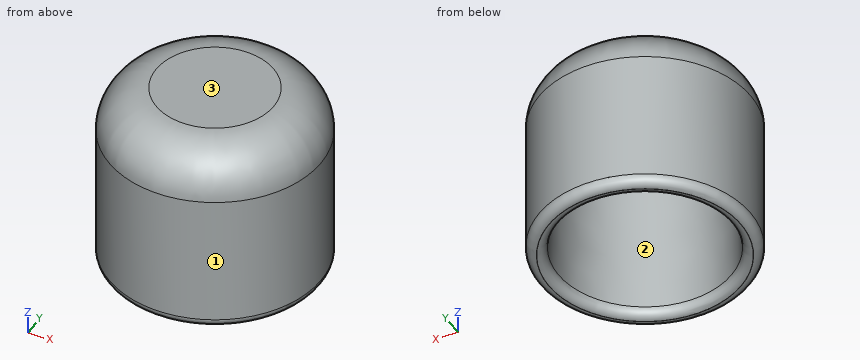
```python
from build123d import *

# Parameters (mm, degrees)
F0_R     = 11.25
F0_R_2   = 9.25
F1_DEPTH = 20
F2_DEPTH = 18
F2_TAPER = 2
F3_R     = 5
F4_R     = 1


with BuildPart() as f1:
    # F0 (on Top) → F1 (new body)
    with BuildSketch(Plane.XY):
        Circle(F0_R)
        Circle(F0_R_2, mode=Mode.SUBTRACT)
        Circle(F0_R_2)
    extrude(amount=F1_DEPTH)

    # F0 (on Top) → F2 (cut)
    with BuildSketch(Plane.XY):
        Circle(F0_R_2)
    extrude(amount=F2_DEPTH, taper=F2_TAPER, mode=Mode.SUBTRACT)

    # F3
    f3_edges = [f1.edges().sort_by_distance(p)[0] for p in [
        (-11.25, 0, 20),
    ]]
    fillet(f3_edges, radius=F3_R)

    # F4
    f4_edges = [f1.edges().sort_by_distance(p)[0] for p in [
        (11.25, 0, 7.5),
        (-11.25, 0, 15),
        (-11.25, 0, 0),
        (-9.25, 0, 0),
        (8.935713, 0, 9),
        (-8.621426, 0, 18),
    ]]
    fillet(f4_edges, radius=F4_R)


solid = f1.part
```
CAD build for the part. Positions are in the model's coordinates, mm. Face numbers are marked on the shaded views. Coordinates: 2 decimals unless noted, no trailing zeros. Order: outer loops, then holes, each group sorted by start corner. A loop starts at its lowest first (then second) coordinate and runs counter-clockwise, first axis right, second up.
(1) Saw through at D-D, the plane z = 3.5. Write the cut outline in (x, y).
Solution:
outline: circle Ø22.5 at (0, 0); hole circle Ø18.26 at (0, 0)
(2) Pin check, flat tips, straight feed: pin 1 Ø8 at (y, z) = (5.5, 16) entering from +X; pin 2 Ø8 at (x, y) = (-3, 4.5) entering from -Z; pin 3 Ø1.5 at (x, z) = (2, 7) entering from -Y. Stop position of each tip, or through.
Solution:
pin 1: stops at x = 11.13
pin 2: stops at z = 0.41
pin 3: stops at y = -11.18
(3) Drill centre lines: L1, parallel to Z at x = -0.5, y = 6; L2, parallel to X at y = -1.25, z = 16.25; L3, parallel to Y at x = 1, z = 1. Where is each one in solid material? Low to high.
Solution:
L1: z = 18 to 20
L2: x = -11.02 to -8.59, 8.59 to 11.02
L3: y = -11.21 to -9.16, 9.16 to 11.21
(4) Mould opens along X. For the marked faces 1, 2 and 3 say: released by +X, released by -X, zero draft, split by the parting line, or undercut.
Solution:
face 1: split by the parting line
face 2: undercut
face 3: zero draft
(5) Saw through at C-C, the plane z = 6.75. Write the cut outline in (x, y).
Solution:
outline: circle Ø22.5 at (0, 0); hole circle Ø18.03 at (0, 0)
